```python
from build123d import *

# Parameters (mm, degrees)
ESQUISSE1_W             = 314
ESQUISSE1_H             = 137
BOSS_EXTRU_1_DEPTH      = 85
ESQUISSE2_W             = 124
ESQUISSE2_H             = 137
ENL_V_MAT_EXTRU_1_DEPTH = 63
ESQUISSE3_W             = 124
ESQUISSE3_H             = 137
ENL_V_MAT_EXTRU_2_DEPTH = 63
ESQUISSE4_W             = 66
ESQUISSE4_H             = 25
ENL_V_MAT_EXTRU_3_DEPTH = 63
ESQUISSE7_W             = 270
ESQUISSE7_H             = 133
ENL_V_MAT_EXTRU_6_DEPTH = 16
ESQUISSE8_W             = 12
ESQUISSE8_H             = 12
ENL_V_MAT_EXTRU_7_DEPTH = 140
ESQUISSE9_W             = 270
ESQUISSE9_H             = 48
ENL_V_MAT_EXTRU_8_DEPTH = 140
ESQUISSE5_W             = 35
ESQUISSE5_H             = 35
ENL_V_MAT_EXTRU_4_DEPTH = 38
ESQUISSE6_W             = 66
ESQUISSE6_H             = 64
ESQUISSE6_W_2           = 47
ESQUISSE6_H_2           = 47
ENL_V_MAT_EXTRU_5_DEPTH = 10
CONG_1_R                = 5
CONG_2_R                = 5


with BuildPart() as part:
    # Esquisse1 → Boss.-Extru.1 (new body)
    with BuildSketch(Plane(origin=(0, 0, 0), x_dir=(1, 0, 0), z_dir=(0, 1, 0))):
        with Locations((157, 68.5)):
            Rectangle(ESQUISSE1_W, ESQUISSE1_H)
    extrude(amount=BOSS_EXTRU_1_DEPTH)

    # Esquisse2 → Enlèv. mat.-Extru.1 (cut)
    with BuildSketch(Plane.XZ):
        with Locations((62, -68.5)):
            Rectangle(ESQUISSE2_W, ESQUISSE2_H)
    extrude(amount=-ENL_V_MAT_EXTRU_1_DEPTH, mode=Mode.SUBTRACT)

    # Esquisse3 → Enlèv. mat.-Extru.2 (cut)
    with BuildSketch(Plane(origin=(0, 0, 0), x_dir=(-1, 0, 0), z_dir=(0, -1, 0))):
        with Locations((-252, 68.5)):
            Rectangle(ESQUISSE3_W, ESQUISSE3_H)
    extrude(amount=-ENL_V_MAT_EXTRU_2_DEPTH, mode=Mode.SUBTRACT)

    # Esquisse4 → Enlèv. mat.-Extru.3 (cut)
    with BuildSketch(Plane.XZ):
        with Locations((157, -124.5)):
            Rectangle(ESQUISSE4_W, ESQUISSE4_H)
    extrude(amount=-ENL_V_MAT_EXTRU_3_DEPTH, mode=Mode.SUBTRACT)

    # Esquisse7 → Enlèv. mat.-Extru.6 (cut)
    with BuildSketch(Plane(origin=(0, 85, 0), x_dir=(1, 0, 0), z_dir=(0, 1, 0))):
        with Locations((157, 66.5)):
            Rectangle(ESQUISSE7_W, ESQUISSE7_H)
    extrude(amount=-ENL_V_MAT_EXTRU_6_DEPTH, mode=Mode.SUBTRACT)

    # Esquisse8 → Enlèv. mat.-Extru.7 (cut)
    with BuildSketch(Plane.XY):
        with Locations((11, 74)):
            Rectangle(ESQUISSE8_W, ESQUISSE8_H)
        with Locations((303, 74)):
            Rectangle(ESQUISSE8_W, ESQUISSE8_H)
    extrude(amount=-ENL_V_MAT_EXTRU_7_DEPTH, mode=Mode.SUBTRACT)

    # Esquisse9 → Enlèv. mat.-Extru.8 (cut)
    with BuildSketch(Plane(origin=(0, 85, 0), x_dir=(1, 0, 0), z_dir=(0, 1, 0))):
        with Locations((157, 24)):
            Rectangle(ESQUISSE9_W, ESQUISSE9_H)
    extrude(amount=-ENL_V_MAT_EXTRU_8_DEPTH, mode=Mode.SUBTRACT)

    # Esquisse5 → Enlèv. mat.-Extru.4 (cut)
    with BuildSketch(Plane.XZ):
        with Locations((157, -80.5)):
            Rectangle(ESQUISSE5_W, ESQUISSE5_H)
    extrude(amount=-ENL_V_MAT_EXTRU_4_DEPTH, mode=Mode.SUBTRACT)

    # Esquisse6 → Enlèv. mat.-Extru.5 (cut)
    with BuildSketch(Plane(origin=(0, 0, 0), x_dir=(-1, 0, 0), z_dir=(0, -1, 0))):
        with Locations((-157, 80)):
            Rectangle(ESQUISSE6_W, ESQUISSE6_H)
        with Locations((-157, 80.5)):
            Rectangle(ESQUISSE6_W_2, ESQUISSE6_H_2, mode=Mode.SUBTRACT)
    extrude(amount=-ENL_V_MAT_EXTRU_5_DEPTH, mode=Mode.SUBTRACT)

    # Congé1
    cong_1_edges = [part.edges().sort_by_distance(p)[0] for p in [
        (180.5, 5, -57),
        (133.5, 5, -57),
        (133.5, 5, -104),
        (180.5, 5, -104),
    ]]
    fillet(cong_1_edges, radius=CONG_1_R)

    # Congé2
    cong_2_edges = [part.edges().sort_by_distance(p)[0] for p in [
        (190, 36.5, -48),
        (124, 36.5, -48),
        (124, 36.5, -112),
        (190, 36.5, -112),
    ]]
    fillet(cong_2_edges, radius=CONG_2_R)


solid = part.part
```
Design review of the part built by this model. Coordinates are the model's own, in mm. A direction names the side the tool comes from. Coordinates: 2 decimals unless noted, no trailing zeros. Order: outer loops, then holes, each group sorted by start corner. A loop starts at its lowest first (then second) coordinate and runs counter-clockwise, first axis right, second up. Notation, with made-up numbers: M 69.25,67 L 99.25,67 A22 cw 99.25,98 Z; hole C 22.5,16.5 d8. An arc over 180 degrees is marked long. Answer as a JSON object with one key per item and string values. Group by question number.
1) Add section D-D, the plane x = 143. Write out the cut boundary in (y, z), then the cut area to 3 significant figures.
2) Tool access review of faces 4 (the flat face through (292, 77, -66)), 5 (the flat face through (157, 10, -52)), 6 (the flat face through (156, 46, -48)), 7 (the flat face through (303, 80, -68)), 8 (the flat face through (157, 36, -112)): name each direction out of +Z, -Z, +X, -X, +Y, -Y from which nothing blocks a thin tool from reaching the whole face with its end or side.
3) Add section C-C, the plane z = -78.5. Write out the cut boundary in (x, y).
4) For pin 1 (11 mm diameter, centred on x = 163, y = 7, fed in from +Z); pin 2 (2 mm diameter, centred on x = 143, z = -76.5, fed in from +Y); pin 3 (13 mm diameter, centred on x = 302.5, z = -95.5, fed in from -Y), all flat-tipped, find the tip position at first contact; note any pin that passes through.
5) Mouldability with a two-part tool opening along X and no side actions: class faces 1 (the flat face through (303, 68, -68)), 2 (the flat face through (0, 74, -68)), 3 (the flat face through (178, 0, -81)) as pulls with the +X half, pulls with the -X half, needs draft (parallel to the pull), parting line crosses it, or undercut.
6) Add section B-B, the plane y = 33. Write out the cut boundary in (x, z), then the cut area to 3 significant figures.
7) Wall thickness on L1, parallel to X at y = 73, z = -77.5; L2, parallel to Z at x = 169, y = 32.5; L3, parallel to X at y = 34, z = -70.5: over which ranges is each line inside the solid? List them lowest first.
8) Add section A-A, the plane z = -14.5. Write out the cut boundary in (x, y).
Computed values:
{
 "1": {"outline": "M 0,-104 L 10,-104 L 10,-112 L 63,-112 L 63,-137 L 85,-137 L 85,-133 L 69,-133 L 69,-48 L 10,-48 L 10,-57 L 0,-57 L 0,-63 L 38,-63 L 38,-98 L 0,-98 Z", "area": "3,130 mm^2"},
 "2": {"face 4": "+Z, +Y", "face 5": "-Y", "face 6": "+Z, +Y, -Y", "face 7": "+Z, -Z", "face 8": "-Z, +X, -X, -Y"},
 "3": {"outline": "M 0,63 L 124,63 L 124,10 L 133.5,10 L 133.5,0 L 139.5,0 L 139.5,38 L 174.5,38 L 174.5,0 L 180.5,0 L 180.5,10 L 190,10 L 190,63 L 314,63 L 314,85 L 292,85 L 292,69 L 22,69 L 22,85 L 0,85 Z; hole M 5,68 L 17,68 L 17,80 L 5,80 Z; hole M 297,68 L 309,68 L 309,80 L 297,80 Z"},
 "4": {"pin 1": "stops at z = -48", "pin 2": "stops at y = 69", "pin 3": "stops at y = 63"},
 "5": {"face 1": "undercut", "face 2": "pulls with the -X half", "face 3": "needs draft"},
 "6": {"outline": "M 124,-107 A5 ccw 129,-112 L 185,-112 A5 ccw 190,-107 L 190,-53 A5 ccw 185,-48 L 129,-48 A5 ccw 124,-53 Z; hole M 139.5,-98 L 174.5,-98 L 174.5,-63 L 139.5,-63 Z", "area": "2,980 mm^2"},
 "7": {"L1": "x = 0 to 5, 17 to 22, 292 to 297, 309 to 314", "L2": "z = -112 to -98, -63 to -48", "L3": "x = 124 to 139.5, 174.5 to 190"},
 "8": {"outline": "M 0,63 L 22,63 L 22,85 L 0,85 Z; M 292,63 L 314,63 L 314,85 L 292,85 Z; hole M 5,68 L 17,68 L 17,80 L 5,80 Z; hole M 297,68 L 309,68 L 309,80 L 297,80 Z"}
}
